Geometry: final body of the model. Coordinates: model frame, mm. A direction names the side the tool comes from. Round coordinates to 2 decimals unless told otherwise and drop trailing zeros. Order: outer loops, then holes, each group sorted by start corner. A loop starts at its lowest first (then second) coordinate and runs counter-clockwise, first axis right, second up. Notation, with made-up numbers: M 65.25,-12 L 88.25,-12 A10 cw 88.25,-3 Z; hole C -22,28 d7. An arc over 180 degrees is marked long. Return JSON: item names as keys, results as strings. Group by question number.
Q1. Access query for faces 1 (the face through (-3, -10.5, 0)), 2 (the face through (9, -10.5, 0)), 3 (the face through (-9, 10.5, 0)). Directions: +Z, -Z, +X, -X, +Y, -Y. A direction counts if a zero-diameter tool reaches every point of the face in a straight line with its end or side. Return the directions, or none.
Q2. Mould query, pull axis Y, two halves, no side actions, for faces 4 (the face through (0, 0, -2.5)), 5 (the face through (5.5, -12, 0)), 6 (the face through (3, 10.5, 0)). Classes: released by +Y, released by -Y, zero draft, split by the parting line, or undercut.
Q3. Cut plane C-C on x = -5.5. Output: boundary loops of the cut face in (y, z), and give its area (4 significant figures).
Q4. Contact query for flat-ended pins moving along their axis: pin 1 (1.5 mm diameter, centred on x = -3, z = 0.5, fed in from -Y); pin 2 (2.5 mm diameter, centred on x = 0.5, z = 1, fed in from +Y). Output: stop coordinate, or through.
Q5. Cut plane B-B on x = 2. Output: boundary loops of the cut face in (y, z).
Q6. Ray query, probe 1 along Y at (x, z) = (8, 0.45); probe 2 along Y at (x, z) = (4.25, -0.65); probe 3 along X at (y, z) = (-10.75, -1.55). Return the intervals inside material, ascending.
Q7. Cut plane A-A on z = 1.7. Output: boundary loops of the cut face in (x, y).
Autodesk Inventor part; units mm, degrees
ref_plane "YZ Plane" through (0, 0, 0) normal (1, 0, 0) x (0, 1, 0)
ref_plane "XZ Plane" through (0, 0, 0) normal (0, 1, 0) x (-1, 0, 0)
ref_plane "XY Plane" through (0, 0, 0) normal (0, 0, 1) x (1, 0, 0)
sketch "Skizze1" plane through (0, 0, 0) normal (0, 0, 1) x (1, 0, 0)
  line L0 (-10.5, 10.5) -> (10.5, 10.5)
  line L1 (10.5, 10.5) -> (10.5, -10.5)
  line L2 (10.5, -10.5) -> (-10.5, -10.5)
  line L3 (-10.5, -10.5) -> (-10.5, 10.5)
  line L4 (-10.5, 10.5) -> (10.5, -10.5) construction
  line L5 (10.5, 10.5) -> (-10.5, -10.5) construction
  point P0 (0, 0)
  dimension "d0" = 21
  dimension "d1" = 21
extrude "Extrusion1" add sketch "Skizze1" along normal mid plane 5
sketch "Skizze2" plane through (0, 0, 2.5) normal (0, 0, 1) x (1, 0, 0)
  line L0 (10.5, 10.5) -> (-10.5, 10.5)
  circle A0 centre (-5.5, 10.5) radius 1.5
  circle A1 centre (5.5, -10.5) radius 1.5
  line L1 (-10.5, -10.5) -> (10.5, -10.5)
  point P0 (0, 0)
  point P1 (0, -10.5)
  point P2 (7, -10.5)
  point P3 (4, -10.5)
  point P4 (-7, 10.5)
  point P5 (-4, 10.5)
  dimension "d4" = 3
  dimension "d5" = 3
  dimension "d6" = 5.5
  dimension "d7" = 5.5
extrude "Extrusion2" add sketch "Skizze2" against normal blind 5 contours L0 A0 | A1 L1 picked at (-5.1257, 11.0709) picked at (5.2587, -11.2635)
properties part number "Kühler"
Result sheet:
{
 "1": {"face 1": "+Z, -Z, -X, -Y", "face 2": "+Z, -Z, +X, -Y", "face 3": "+Z, -Z, -X, +Y"},
 "2": {"face 4": "zero draft", "face 5": "released by -Y", "face 6": "released by +Y"},
 "3": {"outline": "M -10.5,-2.5 L 12,-2.5 L 12,2.5 L -10.5,2.5 Z", "area": "112.5 mm²"},
 "4": {"pin 1": "stops at y = -10.5", "pin 2": "stops at y = 10.5"},
 "5": {"outline": "M -10.5,-2.5 L 10.5,-2.5 L 10.5,2.5 L -10.5,2.5 Z"},
 "6": {"probe 1": "y = -10.5 to 10.5", "probe 2": "y = -11.33 to 10.5", "probe 3": "x = 4.02 to 6.98"},
 "7": {"outline": "M -10.5,-10.5 L 4,-10.5 A1.5 ccw 7,-10.5 L 10.5,-10.5 L 10.5,10.5 L -4,10.5 A1.5 ccw -7,10.5 L -10.5,10.5 Z"}
}
